Drawing for the job (mm, zero at the part's lowest x, y, z). Give positions to 0.01 mm unless a question says otherwise; leave off trailing zeros. Order: outer loops, then holes, each group sorted by start corner. A loop starts at its lowest first (then second) coordinate and runs counter-clockwise, first axis right, second up. Notation, with made-up numbers: (64.5, 89.5) - (80.5, 89.5) arc R17 cw to (80.5, 106.5) - close; hole circle Ø9 at (-29.75, 7.25). An arc over 180 degrees is marked (long way). Use a Markdown table: item, result.
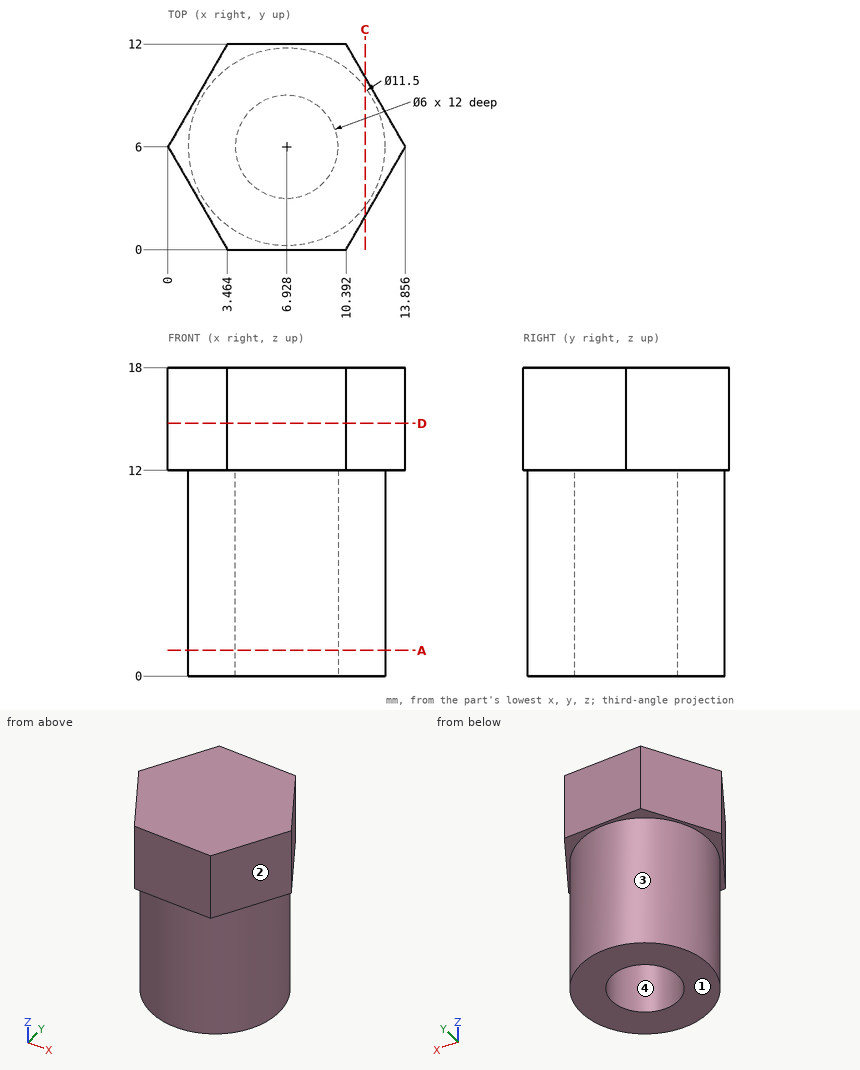
1) Slice it at A-A (z = 1.5). Write the cut outline in (x, y).
Computed:
| item | result |
|---|---|
| outline | circle Ø11.5 at (6.93, 6); hole circle Ø6 at (6.93, 6) |
2) Wall check: line 1 (Z direction, x = 5, y = 5.5); line 2 (Y direction, x = 6.25, z = 8); line 3 (Y direction, x = 9.5, z = 11.25) (1 decimal). Give the ranges that are in metal, low to high. Write a range as from..to.
Computed:
| item | result |
|---|---|
| line 1 | z = 12..18 |
| line 2 | y = 0.29..3.08, 8.92..11.71 |
| line 3 | y = 0.9..4.5, 7.5..11.1 |
3) Slice it at D-D (z = 14.75). Write the cut outline in (x, y).
Computed:
| item | result |
|---|---|
| outline | (0, 6) - (3.46, 0) - (10.39, 0) - (13.86, 6) - (10.39, 12) - (3.46, 12) - close |
4) Two-plate mould, pull along Y, no slides. Class the marked faces 1, 2, 3 and 4: +Y half, -Y half, draft (parallel to the pull), parting line (faces both ways), or undercut.
Computed:
| item | result |
|---|---|
| face 1 | draft |
| face 2 | -Y half |
| face 3 | parting line |
| face 4 | undercut |
5) Pin check, flat tips, straight feed: P1, Ø4, axis at y = 2.5, z = 9.5, coming from the -X side; P2, Ø1, axis at x = 6.5, z = 11, coming from the -Y side; P3, Ø2, axis at y = 3.5, z = 3.5, coming from the +X side. Stop position of each tip, or through.
Computed:
| item | result |
|---|---|
| P1 | stops at x = 1.38 |
| P2 | stops at y = 0.25 |
| P3 | stops at x = 12.48 |
6) Slice it at C-C (x = 11.5). Write the cut outline in (y, z).
Computed:
| item | result |
|---|---|
| outline | (1.92, 12) - (2.51, 12) - (2.51, 0) - (9.49, 0) - (9.49, 12) - (10.08, 12) - (10.08, 18) - (1.92, 18) - close |
